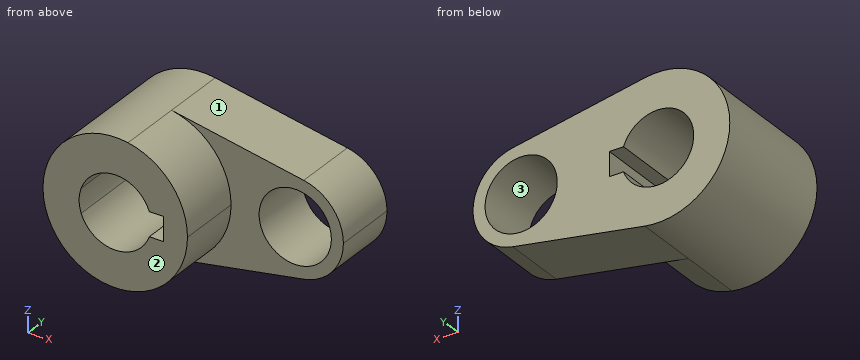
from build123d import *

# Parameters (mm, degrees)
F0_R     = 14.2875
F1_DEPTH = 25.4
F2_DEPTH = 50.8


with BuildPart() as f1:
    # F0 (on Front) → F1 (new body)
    with BuildSketch(Plane.XZ):
        with BuildLine():
            ThreePointArc((5.042647, -28.126541), (21.916025, -18.336262), (28.575, 0))
            ThreePointArc((28.575, 0), (21.916025, 18.336262), (5.042647, 28.126541))
            ThreePointArc((5.042647, 28.126541), (-28.575, 0), (5.042647, -28.126541))
        make_face()
        with BuildLine():
            ThreePointArc((-13.470384, 4.7625), (0, 14.2875), (13.470384, 4.7625))
            Line((13.470384, 4.7625), (19.05, 4.7625))
            Line((19.05, 4.7625), (19.05, -4.7625))
            Line((19.05, -4.7625), (13.470384, -4.7625))
            ThreePointArc((13.470384, -4.7625), (0, -14.2875), (-13.470384, -4.7625))
            Line((-13.470384, -4.7625), (-19.05, -4.7625))
            Line((-19.05, -4.7625), (-19.05, 4.7625))
            Line((-19.05, 4.7625), (-13.470384, 4.7625))
        make_face(mode=Mode.SUBTRACT)
        with BuildLine():
            ThreePointArc((5.042647, 28.126541), (21.916025, 18.336262), (28.575, 0))
            ThreePointArc((28.575, 0), (21.916025, -18.336262), (5.042647, -28.126541))
            Line((5.042647, -28.126541), (57.336765, -18.751028))
            ThreePointArc((57.336765, -18.751028), (34.925, 0), (57.336765, 18.751028))
            Line((57.336765, 18.751028), (5.042647, 28.126541))
        make_face()
        with BuildLine():
            ThreePointArc((73.025, 0), (68.585683, 12.224174), (57.336765, 18.751028))
            ThreePointArc((57.336765, 18.751028), (34.925, 0), (57.336765, -18.751028))
            ThreePointArc((57.336765, -18.751028), (68.585683, -12.224174), (73.025, 0))
        make_face()
        with Locations((53.975, 0)):
            Circle(F0_R, mode=Mode.SUBTRACT)
        with BuildLine():
            ThreePointArc((-13.470384, -4.7625), (-14.2875, 0), (-13.470384, 4.7625))
            Line((-13.470384, 4.7625), (-19.05, 4.7625))
            Line((-19.05, 4.7625), (-19.05, -4.7625))
            Line((-19.05, -4.7625), (-13.470384, -4.7625))
        make_face()
    extrude(amount=F1_DEPTH)

    # F0 (on Front) → F2 (join)
    with BuildSketch(Plane.XZ):
        with BuildLine():
            ThreePointArc((5.042647, -28.126541), (21.916025, -18.336262), (28.575, 0))
            ThreePointArc((28.575, 0), (21.916025, 18.336262), (5.042647, 28.126541))
            ThreePointArc((5.042647, 28.126541), (-28.575, 0), (5.042647, -28.126541))
        make_face()
        with BuildLine():
            ThreePointArc((-13.470384, 4.7625), (0, 14.2875), (13.470384, 4.7625))
            Line((13.470384, 4.7625), (19.05, 4.7625))
            Line((19.05, 4.7625), (19.05, -4.7625))
            Line((19.05, -4.7625), (13.470384, -4.7625))
            ThreePointArc((13.470384, -4.7625), (0, -14.2875), (-13.470384, -4.7625))
            Line((-13.470384, -4.7625), (-19.05, -4.7625))
            Line((-19.05, -4.7625), (-19.05, 4.7625))
            Line((-19.05, 4.7625), (-13.470384, 4.7625))
        make_face(mode=Mode.SUBTRACT)
        with BuildLine():
            ThreePointArc((-13.470384, -4.7625), (-14.2875, 0), (-13.470384, 4.7625))
            Line((-13.470384, 4.7625), (-19.05, 4.7625))
            Line((-19.05, 4.7625), (-19.05, -4.7625))
            Line((-19.05, -4.7625), (-13.470384, -4.7625))
        make_face()
    extrude(amount=F2_DEPTH)


solid = f1.part
For this review, take the finished solid that the model builds, in its own axes (mm). Face numbers are marked on the shaded views. Give positions to 0.01 mm unless a question says otherwise; leave off trailing zeros. Order: outer loops, then holes, each group sorted by start corner. A loop starts at its lowest first (then second) coordinate and runs counter-clockwise, first axis right, second up. Notation, with made-up numbers: (-8.5, 40) - (23.5, 40) arc R18 ccw to (23.5, 61) - close; hole circle Ø2 at (37, 13.5). An arc over 180 degrees is marked (long way). Answer as a JSON object with one key per item and string values. Group by question number.
Item 1: Draft analysis for pull direction X (two halves, no side actions). For the marked faces 1, 2 and 3, state which applies: pulls with the +X half, pulls with the -X half, needs draft (parallel to the pull), parting line crosses it, or undercut.
Item 2: Take a section at B-B on z = -8. Give the boundary of the cut face in (x, y), and give its area (3 significant figures).
Item 3: Take a section at A-A on x = 0. Give the boundary of the cut face in (y, z) (1 decimal), and give its area (3 significant figures).
Item 4: Take a section at D-D on y = -4. Give the number of separate pieces and of enclosed holes in the cut face, and give its area (3 significant figures).
Item 5: Wall thickness on line 1 along X through (y, z) = (-2.5, 5.5); line 2 along Z through (x, y) = (-9, -22); line 3 along Z through (x, y) = (17.5, -12.5): over which ranges is each line inside the solid? List them lowest first.
Item 6: Clearance check with flat-ended pins moving along their axes: pin 1 Ø4.5 at (x, y) = (15.5, -33) entering from +Z; pin 2 Ø12 at (y, z) = (-29, 2.5) entering from -X (3 decimals); pin 3 Ø10 at (x, z) = (35, 3.5) entering from -Y. State where each tip first meets the part, or that it passes through.
Reported:
{
 "1": {"face 1": "pulls with the +X half", "face 2": "needs draft", "face 3": "undercut"},
 "2": {"outline": "(-27.43, -50.8) - (-11.84, -50.8) - (-11.84, 0) - (-27.43, 0) - close; (11.84, -50.8) - (27.43, -50.8) - (27.43, -25.4) - (42.14, -25.4) - (42.14, 0) - (11.84, 0) - close; (65.81, -25.4) - (71.26, -25.4) - (71.26, 0) - (65.81, 0) - close", "area": "2,100 mm^2"},
 "3": {"outline": "(-50.8, -28.6) - (0, -28.6) - (0, -14.3) - (-50.8, -14.3) - close; (-50.8, 14.3) - (0, 14.3) - (0, 28.6) - (-50.8, 28.6) - close", "area": "1,450 mm^2"},
 "4": {"separate pieces": "1", "enclosed holes": "2", "area": "3,130 mm^2"},
 "5": {"line 1": "-28.04 to -13.19, 13.19 to 40.79, 67.16 to 72.21", "line 2": "-27.12 to -11.1, 11.1 to 27.12", "line 3": "-25.89 to -4.76, 4.76 to 25.89"},
 "6": {"pin 1": "z = 25.32", "pin 2": "x = -28.575", "pin 3": "y = -25.4"}
}
